from build123d import *

# Parameters (mm, degrees)
F0_R     = 40
F1_DEPTH = 30


with BuildPart() as f1:
    # F0 (on Front) → F1 (new body)
    with BuildSketch(Plane.XZ):
        with BuildLine():
            Line((70, 10), (49.114953, 10))
            ThreePointArc((49.114953, 10), (49.870079, 5.025321), (50.122636, 0))
            ThreePointArc((50.122636, 0), (49.870079, -5.025321), (49.114953, -10))
            Line((49.114953, -10), (70, -10))
            Line((70, -10), (70, 10))
        make_face()
        with BuildLine():
            ThreePointArc((10, 49.114953), (0, 50.122636), (-10, 49.114953))
            ThreePointArc((-10, 49.114953), (-35.442056, 35.442056), (-49.114953, 10))
            ThreePointArc((-49.114953, 10), (-50.122636, 0), (-49.114953, -10))
            ThreePointArc((-49.114953, -10), (-35.442056, -35.442056), (-10, -49.114953))
            ThreePointArc((-10, -49.114953), (0, -50.122636), (10, -49.114953))
            ThreePointArc((10, -49.114953), (35.442056, -35.442056), (49.114953, -10))
            ThreePointArc((49.114953, -10), (49.870079, -5.025321), (50.122636, 0))
            ThreePointArc((50.122636, 0), (49.870079, 5.025321), (49.114953, 10))
            ThreePointArc((49.114953, 10), (35.442056, 35.442056), (10, 49.114953))
        make_face()
        Circle(F0_R, mode=Mode.SUBTRACT)
        with BuildLine():
            ThreePointArc((-49.114953, -10), (-50.122636, 0), (-49.114953, 10))
            Line((-49.114953, 10), (-70, 10))
            Line((-70, 10), (-70, -10))
            Line((-70, -10), (-49.114953, -10))
        make_face()
        with BuildLine():
            ThreePointArc((10, -49.114953), (0, -50.122636), (-10, -49.114953))
            Line((-10, -49.114953), (-10, -70))
            Line((-10, -70), (10, -70))
            Line((10, -70), (10, -49.114953))
        make_face()
        with BuildLine():
            Line((-5.95824, 70), (-10, 70))
            Line((-10, 70), (-10, 49.114953))
            ThreePointArc((-10, 49.114953), (0, 50.122636), (10, 49.114953))
            Line((10, 49.114953), (10, 70))
            Line((10, 70), (5.95824, 70))
            Line((5.95824, 70), (-5.95824, 70))
        make_face()
        Circle(F0_R)
    extrude(amount=F1_DEPTH)


solid = f1.part
The listing builds one solid part. Answer for the finished solid, in the listing's coordinates (mm). A direction names the side the tool comes from. Round coordinates to 2 decimals unless told otherwise and drop trailing zeros. Write each loop counter-clockwise with the first axis right and the second up, starting at its lowest first coordinate (ties: lowest second). Pieces come first, ordered by that corner, then holes. Notation, with made-up numbers: (20.25, 22) - (71.25, 22) arc R24 ccw to (71.25, 45) - close; hole circle Ø11 at (-4.75, 35). An arc over 180 degrees is marked (long way). Use one line per item in the form item = value. Start each with the question number.
Item 1: Flat-ended cylindrical pins translate along their axes: pin 1 Ø10.5 at (x, y) = (-62, -8.5) entering from +Z; pin 2 Ø2 at (x, y) = (-41, -10) entering from +Z; pin 3 Ø10 at (x, y) = (49.5, -17) entering from -Z. Find the tip coordinate at first contact, or state that the pin passes through.
Item 2: Find the intervals of material crossed by line 1 (Z direction, x = 62.5, y = -23.5); line 2 (X direction, y = -18.5, z = -41), in increasing order. Write a range as [from, to].
Item 3: A cutting plane is placed at C-C (z = 54.5). Write down the section's boundary in (x, y), plus the area to 3 significant figures.
Item 4: A tool of negligible diameter and unlimited length cuts with its end or side. For faces 1 (the flat face through (10, -15, 59)), 2 (the flat face through (59, -15, -10)), 3 (the flat face through (-10, -15, 60)), from which of +Z, -Z, +X, -X, +Y, -Y can it reach the whole face along a straight path? Write none if from no direction.
Item 5: A cutting plane is placed at B-B (x = 52.5). Write down the section's boundary in (y, z).
Item 6: A cutting plane is placed at A-A (y = -6). Write down the section's boundary in (x, z).
The answers:
q1.pin_1 = 10
q1.pin_2 = 30.2
q1.pin_3 = -23.07
q2.line_1 = [-10, 10]
q2.line_2 = [-28.83, 28.83]
q3.outline = (-10, -30) - (10, -30) - (10, 0) - (-10, 0) - close
q3.area = 600 mm^2
q4.face_1 = +Z, +X, +Y, -Y
q4.face_2 = -Z, +X, +Y, -Y
q4.face_3 = +Z, -X, +Y, -Y
q5.outline = (-30, -10) - (0, -10) - (0, 10) - (-30, 10) - close
q6.outline = (-70, -10) - (-49.11, -10) arc R50.12 ccw to (-10, -49.11) - (-10, -70) - (10, -70) - (10, -49.11) arc R50.12 ccw to (49.11, -10) - (70, -10) - (70, 10) - (49.11, 10) arc R50.12 ccw to (10, 49.11) - (10, 70) - (-10, 70) - (-10, 49.11) arc R50.12 ccw to (-49.11, 10) - (-70, 10) - close
